Read the model definition and answer for the solid it produces. Units are mm, in the model's axes. Face numbers are marked on the shaded views. A direction names the side the tool comes from. Round coordinates to 2 decimals unless told otherwise and drop trailing zeros. Write each loop counter-clockwise with the first axis right and the second up, starting at its lowest first coordinate (ties: lowest second). Pieces come first, ordered by that corner, then holes. Notation, with made-up numbers: M 29,-6.75 L 58,-6.75 A21 ccw 58,1.25 Z; hole C 68.5,6 d1. An arc over 180 degrees is marked long. Use one line per item in the form item = value. Start each with the question number.
```python
from build123d import *

# Parameters (mm, degrees)
F0_R     = 9.4996
F1_DEPTH = 19.6596
F2_R     = 2.9845
F3_DEPTH = 12.0396
F4_R     = 2.54
F5_DEPTH = 3.302
F6_W     = 3.175
F6_H     = 3.175
F7_DEPTH = 25.4


with BuildPart() as f1:
    # F0 (on Top) → F1 (new body)
    with BuildSketch(Plane.XY):
        Circle(F0_R)
    extrude(amount=F1_DEPTH)

    # F2 (on face) → F3 (cut)
    with BuildSketch(Plane.XY.offset(19.6596)):
        Circle(F2_R)
    extrude(amount=-F3_DEPTH, mode=Mode.SUBTRACT)

    # F4 (on face) → F5 (join)
    with BuildSketch(Plane.XY.offset(19.6596)):
        with Locations((0, -6.1722)):
            Circle(F4_R)
        with Locations((0, 6.1722)):
            Circle(F4_R)
    extrude(amount=F5_DEPTH)

    # F6 (on face) → F7 (cut)
    with BuildSketch(Plane(origin=(0, 0, 0), x_dir=(1, 0, 0), z_dir=(0, 0, -1))):
        Rectangle(F6_W, F6_H)
    extrude(amount=-F7_DEPTH, mode=Mode.SUBTRACT)


solid = f1.part
```
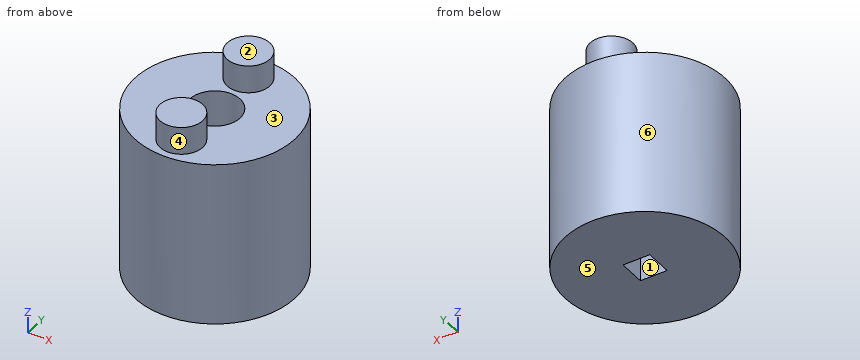
Q1. Find section B-B on y = 0. Write down the section's boundary in (x, z), and give its area (3 significant figures).
Q2. Each of these flat-tipped pins is pushed along its axis until it touches: pin 1 Ø1 at (x, z) = (-5.5, 4) entering from -Y; pin 2 Ø4 at (y, z) = (4.5, 17.5) entering from +X; pin 3 Ø5 at (x, y) = (1, -1) entering from +Z. Where does it stop, or does it pass through?
Q3. Find section A-A on x = 0. Write down the section's boundary in (y, z), and give its area (3 significant figures).
Q4. A tool of negligible diameter and unlimited length cuts with its end or side. For the marked faces 1, 2 and 3, from which of +Z, -Z, +X, -X, +Y, -Y can it reach the whole face along a straight path? Write none if from no direction.
Q5. For a pull along Y with two mould halves and no side action, classify the marked faces 4, 5 and 6 as +Y half, -Y half, draft (parallel to the pull), parting line (faces both ways), or undercut.
Q6. Straight lines are drawn through the part: line 1 (Y direction, x = 0, z = 17); line 2 (Z direction, x = 5.5, y = -6.75); line 3 (X direction, y = -0.5, z = 7.75). For each, find the intervals that lie inside material, in ascending order. Write a range as [from, to].
Q7. Find section C-C on z = 4.75. Write down the section's boundary in (x, y).
Q8. Find section D-D on y = 8. Write down the section's boundary in (x, z), and give its area (3 significant figures).
Response:
q1.outline = M -9.5,0 L -1.59,0 L -1.59,7.62 L -2.98,7.62 L -2.98,19.66 L -9.5,19.66 Z; M 1.59,0 L 9.5,0 L 9.5,19.66 L 2.98,19.66 L 2.98,7.62 L 1.59,7.62 Z
q1.area = 277 mm²
q2.pin_1 = -8.08
q2.pin_2 = 9.16
q2.pin_3 = 19.66
q3.outline = M -9.5,0 L -1.59,0 L -1.59,7.62 L -2.98,7.62 L -2.98,19.66 L -3.63,19.66 L -3.63,22.96 L -8.71,22.96 L -8.71,19.66 L -9.5,19.66 Z; M 1.59,0 L 9.5,0 L 9.5,19.66 L 8.71,19.66 L 8.71,22.96 L 3.63,22.96 L 3.63,19.66 L 2.98,19.66 L 2.98,7.62 L 1.59,7.62 Z
q3.area = 311 mm²
q4.face_1 = +Z, -Z
q4.face_2 = +Z, +X, -X, +Y, -Y
q4.face_3 = +Z
q5.face_4 = undercut
q5.face_5 = draft
q5.face_6 = parting line
q6.line_1 = [-9.5, -2.98], [2.98, 9.5]
q6.line_2 = [0, 19.66]
q6.line_3 = [-9.49, -2.94], [2.94, 9.49]
q7.outline = C 0,0 d19; hole M -1.59,-1.59 L 1.59,-1.59 L 1.59,1.59 L -1.59,1.59 Z
q8.outline = M -5.12,0 L 5.12,0 L 5.12,19.66 L 1.76,19.66 L 1.76,22.96 L -1.76,22.96 L -1.76,19.66 L -5.12,19.66 Z
q8.area = 213 mm²
